Could you check a few things on this model? Use its own coordinates, in mm. Coordinates: 2 decimals unless noted, no trailing zeros. Loops run counter-clockwise (first coordinate to the right, second up) from the corner with the lowest first, then second, coordinate; pieces in that order, holes last. Notation, with made-up numbers: (82, 11.5) - (101, 11.5) arc R26 cw to (101, 41.5) - close; hole circle Ø2 at (13.25, -39.5). An arc over 180 degrees is marked (long way). One line per item, written item: value. Start each with the question number.
(1) If we section it at D-D on y = 1.5: Write out the boundary of the cut face in (x, z), then the cut area to 3 significant figures.
(2) If we section it at A-A on y = 7.5: Write out the boundary of the cut face in (x, z).
(3) If I drill on line 1 along Z through (x, y) = (661.25, 7.5); line 2 along Z through (x, y) = (674.75, 7.5); line 3 along Y through (x, z) = (673.75, 5), over which ranges is the centre line in solid material (lowest first)? Write a range as from..to.
(4) If we mould it in two halves opening along X, with no side actions, what happens to faces 1 (the face through (664.83, 7.395, 58.406)), 2 (the face through (665, 15, 29)), 3 (the face through (668.38, 7.6, 11.89)), 4 (the face through (667.765, 7.605, 43.246))? For each: pulls with the +X half, pulls with the -X half, needs draft (parallel to the pull), parting line crosses it, or undercut.
(5) If we section it at B-B on z = 5: Write out the boundary of the cut face in (x, y).
(6) I'm going to push flat-ended pins straight in: P1, Ø1, axis at y = 13, z = 24.5, coming from the -X side; P2, Ø5, axis at y = 13, z = 9.5, coming from the -X side; P3, Ø2, axis at x = 666.13, z = 43.46, coming from the +Y side; P4, Ø6, axis at y = 13, z = 18, coming from the -X side. Where does each tip first touch, or does it pass through?
(7) If we section it at C-C on x = 657: Write out the boundary of the cut face in (y, z), then the cut area to 3 significant figures.
```python
from build123d import *

# Parameters (mm, degrees)
EXTRUDE_1_DEPTH     = 15
SKETCH_2_R          = 1.45
CUT_EXTRUDE_1_DEPTH = 683.763824452
SKETCH_3_R          = 1.45
CUT_EXTRUDE_2_DEPTH = 69.276600135
SKETCH_4_R          = 1.65
CUT_EXTRUDE_3_DEPTH = 683.763824553
SKETCH_5_R          = 1.65
CUT_EXTRUDE_4_DEPTH = 69.276600157


with BuildPart() as part:
    # 草图1 → 凸台-拉伸1 (new body)
    with BuildSketch(Plane(origin=(0, 0, 0), x_dir=(1, 0, 0), z_dir=(0, 1, 0))):
        Polygon((654.253441162, 0), (650.079202112, -57.331500941), (680, -59.50999899), (680, 0), align=None)
    extrude(amount=EXTRUDE_1_DEPTH)

    # 草图2 → 切除-拉伸1 (cut, through all)
    with BuildSketch(Plane.XZ):
        with Locations(Location((668.307348129, 13.539553134, 0), (0, 0, 270))):
            Circle(SKETCH_2_R)
        with Locations(Location((666.12885008, 43.460351022, 0), (0, 0, 270))):
            Circle(SKETCH_2_R)
    extrude(amount=-CUT_EXTRUDE_1_DEPTH, mode=Mode.SUBTRACT)

    # 草图3 → 切除-拉伸2 (cut, through all)
    with BuildSketch(Plane(origin=(680, 0, 0), x_dir=(0, 0, -1), z_dir=(1, 0, 0))):
        with Locations((-15, 7.5)):
            Circle(SKETCH_3_R)
        with Locations((-5, 7.5)):
            Circle(SKETCH_3_R)
    extrude(amount=-CUT_EXTRUDE_2_DEPTH, mode=Mode.SUBTRACT)

    # 草图4 → 切除-拉伸3 (cut, through all)
    with BuildSketch(Plane(origin=(0, 15, 0), x_dir=(1, 0, 0), z_dir=(0, 1, 0))):
        with Locations(Location((668.307348129, -13.539553134, 0), (0, 0, 270))):
            Circle(SKETCH_4_R)
        with Locations(Location((666.12885008, -43.460351022, 0), (0, 0, 270))):
            Circle(SKETCH_4_R)
    extrude(amount=-CUT_EXTRUDE_3_DEPTH, mode=Mode.SUBTRACT)

    # 草图5 → 切除-拉伸4 (cut, through all)
    with BuildSketch(Plane(origin=(680, 0, 0), x_dir=(0, 0, -1), z_dir=(1, 0, 0))):
        with Locations((-15, 7.5)):
            Circle(SKETCH_5_R)
        with Locations((-5, 7.5)):
            Circle(SKETCH_5_R)
    extrude(amount=-CUT_EXTRUDE_4_DEPTH, mode=Mode.SUBTRACT)


solid = part.part
```
Values:
1. outline: (650.08, 57.33) - (654.25, 0) - (680, 0) - (680, 59.51) - close; hole circle Ø3.3 at (666.13, 43.46); hole circle Ø3.3 at (668.31, 13.54)
1. area: 1,610 mm2
2. outline: (650.08, 57.33) - (653.04, 16.65) - (680, 16.65) - (680, 59.51) - close; (653.28, 13.35) - (653.77, 6.65) - (680, 6.65) - (680, 13.35) - (669.95, 13.35) arc R1.65 cw to (666.67, 13.35) - close; (654.01, 3.35) - (654.25, 0) - (680, 0) - (680, 3.35) - close; hole circle Ø3.3 at (666.13, 43.46)
3. line 1: z = 0..3.35, 6.65..13.35, 16.65..58.14
3. line 2: z = 0..3.35, 6.65..13.35, 16.65..59.13
3. line 3: y = 0..5.85, 9.15..15
4. face 1: pulls with the -X half
4. face 2: needs draft
4. face 3: undercut
4. face 4: undercut
5. outline: (653.89, 0) - (680, 0) - (680, 5.85) - (653.89, 5.85) - close; (653.89, 9.15) - (680, 9.15) - (680, 15) - (653.89, 15) - close
6. P1: stops at x = 652.43
6. P2: stops at x = 653.38
6. P3: passes through
6. P4: stops at x = 652.72
7. outline: (0, 0) - (15, 0) - (15, 57.84) - (0, 57.84) - close; hole circle Ø3.3 at (7.5, 5); hole circle Ø3.3 at (7.5, 15)
7. area: 850 mm2
